Autodesk Inventor part; units mm, degrees
ref_plane "YZ Plane" through (0, 0, 0) normal (1, 0, 0) x (0, 1, 0)
ref_plane "XZ Plane" through (0, 0, 0) normal (0, 1, 0) x (-1, 0, 0)
ref_plane "XY Plane" through (0, 0, 0) normal (0, 0, 1) x (1, 0, 0)
sketch "Sketch1" plane through (0, 0, 0) normal (0, 0, 1) x (1, 0, 0)
  line L0 (0, 0) -> (78.74, 0)
  line L1 (78.74, 0) -> (78.74, -58.42)
  line L2 (78.74, -58.42) -> (0, -58.42)
  line L3 (0, -58.42) -> (0, 0)
  dimension "d0" = 78.74
  dimension "d1" = 58.42
extrude "Extrusion1" add sketch "Sketch1" along normal blind 17.78
fillet "Fillet1" radius 6.35 2 edges at (78.74, -29.21, 17.78) (0, -29.21, 17.78)
sketch "Sketch2" plane through (0, 0, 0) normal (0, 0, -1) x (-1, 0, 0)
  circle A0 centre (-69.85, -29.21) radius 1.5875
  line L0 (-78.74, 0) -> (-78.74, -58.42)
  line L1 (0, 0) -> (-78.74, 0)
  circle A1 centre (-8.89, -29.21) radius 1.5875
  line L2 (0, -58.42) -> (0, 0)
  dimension "d5" = 3.175
  dimension "d6" = 8.89
  dimension "d7" = 29.21
  dimension "d8" = 3.175
  dimension "d9" = 8.89
extrude "Extrusion2" cut sketch "Sketch2" against normal blind 25.4
sketch "Sketch3" plane through (0, 0, 17.78) normal (0, 0, 1) x (1, 0, 0)
  line L0 (6.35, -58.42) -> (6.35, 0)
  line L1 (72.39, 0) -> (72.39, -58.42)
  line L2 (6.35, -5.08) -> (72.39, -5.08)
  line L3 (72.39, -5.08) -> (72.39, -53.34)
  line L4 (72.39, -53.34) -> (6.35, -53.34)
  line L5 (6.35, -53.34) -> (6.35, -5.08)
  line L6 (72.39, 0) -> (6.35, 0)
  line L7 (6.35, -58.42) -> (72.39, -58.42)
  point P0 (0, 0)
  dimension "d12" = 5.08
  dimension "d13" = 5.08
extrude "Extrusion3" cut sketch "Sketch3" against normal blind 12.7 contours L0 L2 L1 L4
properties part number "BatteryHolder" material "ABS Plastic"
Part model, mm, in its own coordinate system. A direction names the side the tool comes from. Give positions to 0.01 mm unless a question says otherwise; leave off trailing zeros. Write each loop counter-clockwise with the first axis right and the second up, starting at its lowest first coordinate (ties: lowest second). Pieces come first, ordered by that corner, then holes. Notation, with made-up numbers: M 76,32.25 L 100,32.25 A12 cw 100,36.25 Z; hole C 6,33.25 d3. An arc over 180 degrees is marked long. Use CSV: the item, a comma, the result in double quotes.
Item 1: Pull direction X, two halves, no side cores. Call faces 3 (the face through (40, -53.34, 12)), 4 (the face through (39, -3, 17.78)), 5 (the face through (0, -30, 6)): +X half, -X half, draft (parallel to the pull), parting line (faces both ways), or undercut.
Taken from the geometry:
face 3,"undercut"
face 4,"draft"
face 5,"-X half"
Item 2: Slice it at A-A on y = -29.21. Write the cut outline in (x, z), plus the area to 3 significant figures.
Taken from the geometry:
outline,"M 0,0 L 7.3,0 L 7.3,5.08 L 6.35,5.08 L 6.35,17.78 A6.35 ccw 0,11.43 Z; M 10.48,0 L 68.26,0 L 68.26,5.08 L 10.48,5.08 Z; M 71.44,0 L 78.74,0 L 78.74,11.43 A6.35 ccw 72.39,17.78 L 72.39,5.08 L 71.44,5.08 Z"
area,"512 mm²"
Item 3: Which spindle directions (+Z, -Z, +X, -X, +Y, -Y) get a long thin tool onto all of the face, cutting with end or side? Do faces 1 (the face through (1.81, -28.8, 15.87)), 2 (the face through (72.39, -29, 12)). Say none if no direction does.
Taken from the geometry:
face 1,"+Z, -X, +Y, -Y"
face 2,"+Z"
Item 4: Pin check, flat tips, straight feed: P1, Ø2.5, axis at x = 8.89, y = -29.21, coming from the +Z side; P2, Ø3, axis at y = -8, z = 15.5, coming from the -X side. Stop position of each tip, or through.
Taken from the geometry:
P1,"passes through"
P2,"stops at x = 0.54"
Item 5: Drill centre lines: probe 1 along X at (y, z) = (-8, 8.75); probe 2 along Y at (x, z) = (69.85, 3.65); probe 3 along Y at (x, z) = (30.5, 5.25). Where is each one in solid material? Low to high.
Taken from the geometry:
probe 1,"x = 0 to 6.35, 72.39 to 78.74"
probe 2,"y = -58.42 to -30.8, -27.62 to 0"
probe 3,"y = -58.42 to -53.34, -5.08 to 0"
Item 6: Slice it at B-B on x = 8.89. Write the cut outline in (y, z), plus the area to 3 significant figures.
Taken from the geometry:
outline,"M -58.42,0 L -30.8,0 L -30.8,5.08 L -53.34,5.08 L -53.34,17.78 L -58.42,17.78 Z; M -27.62,0 L 0,0 L 0,17.78 L -5.08,17.78 L -5.08,5.08 L -27.62,5.08 Z"
area,"410 mm²"
Item 7: Slice it at C-C on z = 14.75. Write the cut outline in (x, y).
Taken from the geometry:
outline,"M 0.94,-58.42 L 77.8,-58.42 L 77.8,0 L 0.94,0 Z; hole M 6.35,-53.34 L 72.39,-53.34 L 72.39,-5.08 L 6.35,-5.08 Z"
Item 8: Slice it at D-D on y = -38.5. Write the cut outline in (x, z).
Taken from the geometry:
outline,"M 0,0 L 78.74,0 L 78.74,11.43 A6.35 ccw 72.39,17.78 L 72.39,5.08 L 6.35,5.08 L 6.35,17.78 A6.35 ccw 0,11.43 Z"
